```python
from build123d import *

# Parameters (mm, degrees)
F0_R     = 11.5110265847
F0_R_2   = 11.2157876958
F1_DEPTH = 25.4
F2_DEPTH = 25.4


with BuildPart() as f1:
    # F0 (on Front) → F1 (new body)
    with BuildSketch(Plane.XZ):
        with BuildLine():
            add(Edge.make_bspline(
                [(-42.6191106401, -9.9153485832), (-20.6350689987, -21.9972569119), (7.738026744, -31.8239785263), (29.3943516136, -32.4141145567)],
                knots=[0.8430854965, 0.8430854965, 0.8430854965, 0.8430854965, 1, 1, 1, 1], degree=3))
            ThreePointArc((29.3943516136, -32.4141145567), (40.0057537744, -17.7268833761), (43.7573162944, 0))
            ThreePointArc((43.7573162944, 0), (37.9839654581, 21.7237450123), (22.1873875452, 37.715017741))
            add(Edge.make_bspline(
                [(22.1873875452, 37.715017741), (11.6721202081, 40.2099582819), (-0.1429108616, 41.6665900381), (-11.8526616126, 42.1214570259)],
                knots=[0.4240545667, 0.4240545667, 0.4240545667, 0.4240545667, 0.4970480989, 0.4970480989, 0.4970480989, 0.4970480989], degree=3))
            ThreePointArc((-11.8526616126, 42.1214570259), (-37.6663082553, 22.2699787089), (-42.6191106402, -9.9153485832))
        make_face()
        with Locations((-27.6805255562, 3.7134094164)):
            Circle(F0_R, mode=Mode.SUBTRACT)
        with Locations((16.7762394994, -8.2583986223)):
            Circle(F0_R_2, mode=Mode.SUBTRACT)
        with BuildLine():
            add(Edge.make_bspline(
                [(-42.7234657978, 40.8730333774), (-61.8148502648, 38.3753901199), (-91.4828084934, 26.3670705011), (-62.8281013178, 1.1910337993), (-42.6191106401, -9.9153485832)],
                knots=[0.5639979758, 0.5639979758, 0.5639979758, 0.5639979758, 0.6988406943, 0.8430854965, 0.8430854965, 0.8430854965, 0.8430854965], degree=3))
            ThreePointArc((-42.6191106402, -9.9153485832), (-37.6663082553, 22.2699787089), (-11.8526616126, 42.1214570259))
            add(Edge.make_bspline(
                [(-11.8526616126, 42.1214570259), (-22.5928785611, 42.5386623307), (-33.2445272732, 42.1131219072), (-42.7234657978, 40.8730333774)],
                knots=[0.4970480989, 0.4970480989, 0.4970480989, 0.4970480989, 0.5639979758, 0.5639979758, 0.5639979758, 0.5639979758], degree=3))
        make_face()
        with BuildLine():
            ThreePointArc((43.7573162944, 0), (40.0057537744, -17.7268833761), (29.3943516136, -32.4141145567))
            add(Edge.make_bspline(
                [(29.3943516136, -32.4141145567), (56.9711731435, -33.1655844432), (84.9977641322, -9.2707192189), (67.106763708, 16.3997179852), (54.1769252073, 24.7250533856)],
                knots=[0, 0, 0, 0, 0.1998124467, 0.3356238703, 0.3356238703, 0.3356238703, 0.3356238703], degree=3))
            add(Edge.make_bspline(
                [(54.1769252073, 24.7250533856), (45.7579380993, 30.1459170261), (34.9264945205, 34.6924303516), (22.1873875452, 37.715017741)],
                knots=[0.3356238703, 0.3356238703, 0.3356238703, 0.3356238703, 0.4240545667, 0.4240545667, 0.4240545667, 0.4240545667], degree=3))
            ThreePointArc((22.1873875452, 37.715017741), (37.9839654581, 21.7237450123), (43.7573162944, 0))
        make_face()
    extrude(amount=F1_DEPTH)

    # F0 (on Front) → F2 (join)
    with BuildSketch(Plane.XZ):
        with BuildLine():
            add(Edge.make_bspline(
                [(-42.6191106401, -9.9153485832), (-20.6350689987, -21.9972569119), (7.738026744, -31.8239785263), (29.3943516136, -32.4141145567)],
                knots=[0.8430854965, 0.8430854965, 0.8430854965, 0.8430854965, 1, 1, 1, 1], degree=3))
            ThreePointArc((29.3943516136, -32.4141145567), (40.0057537744, -17.7268833761), (43.7573162944, 0))
            ThreePointArc((43.7573162944, 0), (37.9839654581, 21.7237450123), (22.1873875452, 37.715017741))
            add(Edge.make_bspline(
                [(22.1873875452, 37.715017741), (11.6721202081, 40.2099582819), (-0.1429108616, 41.6665900381), (-11.8526616126, 42.1214570259)],
                knots=[0.4240545667, 0.4240545667, 0.4240545667, 0.4240545667, 0.4970480989, 0.4970480989, 0.4970480989, 0.4970480989], degree=3))
            ThreePointArc((-11.8526616126, 42.1214570259), (-37.6663082553, 22.2699787089), (-42.6191106402, -9.9153485832))
        make_face()
        with Locations((-27.6805255562, 3.7134094164)):
            Circle(F0_R, mode=Mode.SUBTRACT)
        with Locations((16.7762394994, -8.2583986223)):
            Circle(F0_R_2, mode=Mode.SUBTRACT)
        with BuildLine():
            ThreePointArc((43.7573162944, 0), (40.0057537744, -17.7268833761), (29.3943516136, -32.4141145567))
            add(Edge.make_bspline(
                [(29.3943516136, -32.4141145567), (56.9711731435, -33.1655844432), (84.9977641322, -9.2707192189), (67.106763708, 16.3997179852), (54.1769252073, 24.7250533856)],
                knots=[0, 0, 0, 0, 0.1998124467, 0.3356238703, 0.3356238703, 0.3356238703, 0.3356238703], degree=3))
            add(Edge.make_bspline(
                [(54.1769252073, 24.7250533856), (45.7579380993, 30.1459170261), (34.9264945205, 34.6924303516), (22.1873875452, 37.715017741)],
                knots=[0.3356238703, 0.3356238703, 0.3356238703, 0.3356238703, 0.4240545667, 0.4240545667, 0.4240545667, 0.4240545667], degree=3))
            ThreePointArc((22.1873875452, 37.715017741), (37.9839654581, 21.7237450123), (43.7573162944, 0))
        make_face()
        with BuildLine():
            ThreePointArc((-42.6191106402, -9.9153485832), (-13.0488382782, -41.7663806054), (29.3943516136, -32.4141145567))
            add(Edge.make_bspline(
                [(-42.6191106401, -9.9153485832), (-20.6350689987, -21.9972569119), (7.738026744, -31.8239785263), (29.3943516136, -32.4141145567)],
                knots=[0.8430854965, 0.8430854965, 0.8430854965, 0.8430854965, 1, 1, 1, 1], degree=3))
        make_face()
        with BuildLine():
            add(Edge.make_bspline(
                [(-42.7234657978, 40.8730333774), (-61.8148502648, 38.3753901199), (-91.4828084934, 26.3670705011), (-62.8281013178, 1.1910337993), (-42.6191106401, -9.9153485832)],
                knots=[0.5639979758, 0.5639979758, 0.5639979758, 0.5639979758, 0.6988406943, 0.8430854965, 0.8430854965, 0.8430854965, 0.8430854965], degree=3))
            ThreePointArc((-42.6191106402, -9.9153485832), (-37.6663082553, 22.2699787089), (-11.8526616126, 42.1214570259))
            add(Edge.make_bspline(
                [(-11.8526616126, 42.1214570259), (-22.5928785611, 42.5386623307), (-33.2445272732, 42.1131219072), (-42.7234657978, 40.8730333774)],
                knots=[0.4970480989, 0.4970480989, 0.4970480989, 0.4970480989, 0.5639979758, 0.5639979758, 0.5639979758, 0.5639979758], degree=3))
        make_face()
        with BuildLine():
            add(Edge.make_bspline(
                [(54.1769252073, 24.7250533856), (45.7579380993, 30.1459170261), (34.9264945205, 34.6924303516), (22.1873875452, 37.715017741)],
                knots=[0.3356238703, 0.3356238703, 0.3356238703, 0.3356238703, 0.4240545667, 0.4240545667, 0.4240545667, 0.4240545667], degree=3))
            ThreePointArc((54.1769252073, 24.7250533856), (8.8421199016, 51.4937982895), (-42.7234657978, 40.8730333774))
            add(Edge.make_bspline(
                [(-11.8526616126, 42.1214570259), (-22.5928785611, 42.5386623307), (-33.2445272732, 42.1131219072), (-42.7234657978, 40.8730333774)],
                knots=[0.4970480989, 0.4970480989, 0.4970480989, 0.4970480989, 0.5639979758, 0.5639979758, 0.5639979758, 0.5639979758], degree=3))
            ThreePointArc((-11.8526616126, 42.1214570259), (5.6174564367, 43.3952406661), (22.1873875452, 37.715017741))
        make_face()
    extrude(amount=F2_DEPTH)


solid = f1.part
```
The listing builds one solid part. Answer for the finished solid, in the listing's coordinates (mm). Coordinates: 2 decimals unless noted, no trailing zeros. Loops run counter-clockwise (first coordinate to the right, second up) from the corner with the lowest first, then second, coordinate; pieces in that order, holes last. Notation, with made-up numbers: (89.25, 13.5) - (105.25, 13.5) arc R13 ccw to (105.25, 32.5) - close; hole circle Ø7 at (28, -28). An arc over 180 degrees is marked (long way). Use a Markdown table: item, result. Add a question column.
1) The mould has two halves that part along X. Classify faces 1 (the cylindrical face through (9.585, -12.522, 51.366)), 2 (the cylindrical face through (-17.05, -12.52, -0.7)), 3 (the flat face through (-4, -25.4, 5)): released by +X, released by -X, zero draft, split by the parting line, or undercut.
2) The part is cut by section B-B, the plane z = -35.5. Give the vertices of the cut face in (x, y).
3) Given pin 1 (5 mm diameter, centred on x = -1, y = -13.5, fed in from +Z); pin 2 (10 mm diameter, centred on y = -13.5, z = 28.5, fed in from +X); pin 3 (6 mm diameter, centred on x = 13, y = -4, fed in from -Z), each flat-ended and moving along its own axis, determine where each tip first touches the part or whether it passes through.
4) Find the intervals of material crossed by line 1 (Z direction, x = 20, y = -7.5); line 2 (X direction, y = -17, z = -5); line 3 (X direction, y = -12.75, z = -17.5), in increasing order.
5) The part is cut by section A-A, the plane x = 18.5. State how many separate pieces and enclosed holes the cut face has, and give its area (3 significant figures).
Here are the results:
| question | item | result |
|---|---|---|
| 1 | face 1 | split by the parting line |
| 1 | face 2 | undercut |
| 1 | face 3 | zero draft |
| 2 | outline | (-25.58, -25.4) - (25.58, -25.4) - (25.58, 0) - (-25.58, 0) - close |
| 3 | pin 1 | stops at z = 52.49 |
| 3 | pin 2 | stops at x = 56.02 |
| 3 | pin 3 | stops at z = -42.6 |
| 4 | line 1 | z = -38.92 to -19, 2.48 to 38.22, 38.92 to 48.72 |
| 4 | line 2 | x = -51.01 to -35.2, -20.16 to 6.04, 27.51 to 74.02 |
| 4 | line 3 | x = -40.11 to 10.42, 23.13 to 68.99 |
| 5 | separate pieces | 3 |
| 5 | enclosed holes | 0 |
| 5 | area | 1,670 mm^2 |
